The listing builds one solid part. Answer for the finished solid, in the listing's coordinates (mm). A direction names the side the tool comes from. Give positions to 0.01 mm unless a question says otherwise; leave off trailing zeros. Write each loop counter-clockwise with the first axis right and the second up, starting at its lowest first coordinate (ties: lowest second). Pieces come first, ordered by that corner, then holes. Notation, with made-up numbers: M 65.25,-9 L 84.25,-9 A12 ccw 84.25,-3 Z; hole C 80.25,10.5 d3. An arc over 180 degrees is marked long. Answer as a JSON object with one key per item and string values.
```python
from build123d import *

# Parameters (mm, degrees)
EXTRUSION1_DEPTH             = 48
ENL_V_MAT_EXTRU_1_DEPTH      = 97
R_P_TITION_CIRCULAIRE1_COUNT = 4


with BuildPart() as part:
    # Esquisse1 → Extrusion1 (new body, symmetric)
    with BuildSketch(Plane.XY):
        with BuildLine():
            Line((-6, 5), (-6, -5))
            ThreePointArc((-6, -5), (-5.707106781, -5.707106781), (-5, -6))
            Line((-5, -6), (5, -6))
            ThreePointArc((5, -6), (5.707106781, -5.707106781), (6, -5))
            Line((6, -5), (6, 5))
            ThreePointArc((6, 5), (5.707106781, 5.707106781), (5, 6))
            Line((5, 6), (-5, 6))
            ThreePointArc((-5, 6), (-5.707106781, 5.707106781), (-6, 5))
        make_face()
    extrude(amount=EXTRUSION1_DEPTH, both=True)

    # Esquisse3 → Enl_v. mat.-Extru.1 (cut, through all)
    with BuildSketch(Plane.XY.offset(48)):
        Polygon((6, 2), (4.8, 2), (4.8, 4), (2, 1), (2, -1), (4.8, -4), (4.8, -2), (6, -2), align=None)
    enl_v_mat_extru_1 = extrude(amount=-ENL_V_MAT_EXTRU_1_DEPTH, mode=Mode.SUBTRACT)

    # R_p_tition circulaire1: Enl_v. mat.-Extru.1 ×4 about axis
    r_p_tition_circulaire1_axis = Axis((0, 0, 0), (0, 0, 1))
    for i in range(1, R_P_TITION_CIRCULAIRE1_COUNT):
        add(enl_v_mat_extru_1.rotate(r_p_tition_circulaire1_axis, i * 360 / R_P_TITION_CIRCULAIRE1_COUNT), mode=Mode.SUBTRACT)


solid = part.part
```
1. A cutting plane is placed at A-A, the plane x = 0. Give the vertices of the cut face in (y, z).
Verdict:
{"outline": "M -2,-48 L 2,-48 L 2,48 L -2,48 Z"}
2. Consider line 1 along X through (y, z) = (2.75, -5); line 2 along Y through (x, z) = (2.5, -18); line 3 along X through (y, z) = (-3.5, -23). Determine where each line is inside the solid, lowest interval first.
Verdict:
{"line 1": "x = -6 to -4.8, -3.63 to -1.8, 1.8 to 3.63, 4.8 to 6", "line 2": "y = -6 to -4.8, -3.4 to -1.54, 1.54 to 3.4, 4.8 to 6", "line 3": "x = -6 to -4.8, -4.33 to -2.61, 2.61 to 4.33, 4.8 to 6"}
3. The mould has two halves that part along Y. Classify faces 5 (the flat face through (6, 3, 1)), 6 (the flat face through (-3, 6, 1)), 7 (the flat face through (3, -4.8, 1)): released by +Y, released by -Y, zero draft, split by the parting line, or undercut.
Verdict:
{"face 5": "zero draft", "face 6": "released by +Y", "face 7": "undercut"}
4. For faces 1 (the flat face through (0, -2, 1)), 2 (the flat face through (4, 6, 1)), 3 (the flat face through (2, 0, 1)), 4 (the flat face through (0, 2, 1)), determine the directions among +Z, -Z, +X, -X, +Y, -Y from which every point of the face is accessible in a straight line to the end or side of a thin tool.
Verdict:
{"face 1": "+Z, -Z, -Y", "face 2": "+Z, -Z, +X, -X, +Y", "face 3": "+Z, -Z, +X", "face 4": "+Z, -Z, +Y"}
5. Flat-ended cylindrical pins translate along their axes: pin 1 (1.5 mm diameter, centred on y = 0.5, z = 20, fed in from +X); pin 2 (0.6 mm diameter, centred on x = 5.5, z = 1.5, fed in from +Y); pin 3 (1.6 mm diameter, centred on y = -0.5, z = 21, fed in from -X). Find the tip coordinate at first contact, or state that the pin passes through.
Verdict:
{"pin 1": "stops at x = 2.23", "pin 2": "stops at y = 5.98", "pin 3": "stops at x = -2.28"}
